from build123d import *

# Parameters (mm, degrees)
F0_R     = 175
F0_R_2   = 13
F1_DEPTH = 4


with BuildPart() as f1:
    # F0 (on Top) → F1 (new body)
    with BuildSketch(Plane.XY):
        Circle(F0_R)
        with Locations((-107.480231, -107.480231)):
            Circle(F0_R_2, mode=Mode.SUBTRACT)
        with Locations((-76, -131.635861)):
            Circle(F0_R_2, mode=Mode.SUBTRACT)
        with Locations((-39.340495, -146.820726)):
            Circle(F0_R_2, mode=Mode.SUBTRACT)
        with Locations((-45.922012, -110.865544)):
            Circle(F0_R_2, mode=Mode.SUBTRACT)
        with Locations((-73.051371, -95.202401)):
            Circle(F0_R_2, mode=Mode.SUBTRACT)
        with Locations((-15.663143, -118.973383)):
            Circle(F0_R_2, mode=Mode.SUBTRACT)
        with Locations((-131.635861, -76)):
            Circle(F0_R_2, mode=Mode.SUBTRACT)
        with Locations((-95.202401, -73.051371)):
            Circle(F0_R_2, mode=Mode.SUBTRACT)
        with Locations((-110.865544, -45.922012)):
            Circle(F0_R_2, mode=Mode.SUBTRACT)
        with Locations((-146.820726, -39.340495)):
            Circle(F0_R_2, mode=Mode.SUBTRACT)
        with Locations((-118.973383, -15.663143)):
            Circle(F0_R_2, mode=Mode.SUBTRACT)
        with Locations((0, -152)):
            Circle(F0_R_2, mode=Mode.SUBTRACT)
        with Locations((39.340495, -146.820726)):
            Circle(F0_R_2, mode=Mode.SUBTRACT)
        with Locations((76, -131.635861)):
            Circle(F0_R_2, mode=Mode.SUBTRACT)
        with Locations((15.663143, -118.973383)):
            Circle(F0_R_2, mode=Mode.SUBTRACT)
        with Locations((45.922012, -110.865544)):
            Circle(F0_R_2, mode=Mode.SUBTRACT)
        with Locations((73.051371, -95.202401)):
            Circle(F0_R_2, mode=Mode.SUBTRACT)
        with Locations((107.480231, -107.480231)):
            Circle(F0_R_2, mode=Mode.SUBTRACT)
        with Locations((95.202401, -73.051371)):
            Circle(F0_R_2, mode=Mode.SUBTRACT)
        with Locations((110.865544, -45.922012)):
            Circle(F0_R_2, mode=Mode.SUBTRACT)
        with Locations((131.635861, -76)):
            Circle(F0_R_2, mode=Mode.SUBTRACT)
        with Locations((118.973383, -15.663143)):
            Circle(F0_R_2, mode=Mode.SUBTRACT)
        with Locations((146.820726, -39.340495)):
            Circle(F0_R_2, mode=Mode.SUBTRACT)
        with Locations((-152, 0)):
            Circle(F0_R_2, mode=Mode.SUBTRACT)
        with Locations((-146.820726, 39.340495)):
            Circle(F0_R_2, mode=Mode.SUBTRACT)
        with Locations((-118.973383, 15.663143)):
            Circle(F0_R_2, mode=Mode.SUBTRACT)
        with Locations((-131.635861, 76)):
            Circle(F0_R_2, mode=Mode.SUBTRACT)
        with Locations((-110.865544, 45.922012)):
            Circle(F0_R_2, mode=Mode.SUBTRACT)
        with Locations((-95.202401, 73.051371)):
            Circle(F0_R_2, mode=Mode.SUBTRACT)
        with Locations((-107.480231, 107.480231)):
            Circle(F0_R_2, mode=Mode.SUBTRACT)
        with Locations((-73.051371, 95.202401)):
            Circle(F0_R_2, mode=Mode.SUBTRACT)
        with Locations((-45.922012, 110.865544)):
            Circle(F0_R_2, mode=Mode.SUBTRACT)
        with Locations((-15.663143, 118.973383)):
            Circle(F0_R_2, mode=Mode.SUBTRACT)
        with Locations((-76, 131.635861)):
            Circle(F0_R_2, mode=Mode.SUBTRACT)
        with Locations((-39.340495, 146.820726)):
            Circle(F0_R_2, mode=Mode.SUBTRACT)
        with Locations((118.973383, 15.663143)):
            Circle(F0_R_2, mode=Mode.SUBTRACT)
        with Locations((152, 0)):
            Circle(F0_R_2, mode=Mode.SUBTRACT)
        with Locations((146.820726, 39.340495)):
            Circle(F0_R_2, mode=Mode.SUBTRACT)
        with Locations((110.865544, 45.922012)):
            Circle(F0_R_2, mode=Mode.SUBTRACT)
        with Locations((95.202401, 73.051371)):
            Circle(F0_R_2, mode=Mode.SUBTRACT)
        with Locations((131.635861, 76)):
            Circle(F0_R_2, mode=Mode.SUBTRACT)
        with Locations((15.663143, 118.973383)):
            Circle(F0_R_2, mode=Mode.SUBTRACT)
        with Locations((73.051371, 95.202401)):
            Circle(F0_R_2, mode=Mode.SUBTRACT)
        with Locations((45.922012, 110.865544)):
            Circle(F0_R_2, mode=Mode.SUBTRACT)
        with Locations((0, 152)):
            Circle(F0_R_2, mode=Mode.SUBTRACT)
        with Locations((39.340495, 146.820726)):
            Circle(F0_R_2, mode=Mode.SUBTRACT)
        with Locations((76, 131.635861)):
            Circle(F0_R_2, mode=Mode.SUBTRACT)
        with Locations((107.480231, 107.480231)):
            Circle(F0_R_2, mode=Mode.SUBTRACT)
    extrude(amount=F1_DEPTH)


solid = f1.part
Geometry check sheet. Reference: the model listing, model coordinates, mm. Round coordinates to 2 decimals unless told otherwise and drop trailing zeros. Loops run counter-clockwise (first coordinate to the right, second up) from the corner with the lowest first, then second, coordinate; pieces in that order, holes last.
Item 1: Thickness scan on line 1 (Y direction, x = -136, z = 1.3); line 2 (X direction, y = 11.5, z = 2.9); line 3 (Y direction, x = -94, z = 2.25). Record the ranges inside material, lowest first.
Item 2: Cross-section at A-A on x = 69.5. Record the boundary of the cut face in (y, z), then the cut area to 3 significant figures.
Item 3: Gauge pin test, flat ends, axial feed: pin 1 (1.5 mm diameter, centred on y = 101, z = 2, fed in from +X); pin 2 (4 mm diameter, centred on x = 134, y = -50.5, fed in from -Z). Record the tip position at first contact, or that the pin passes through.
Item 4: Mould release check, pull along X, two halves, no side actions. Record for faces 1 (the cylindrical face through (-128.982, 118.273, 1.972)), 2 (the cylindrical face through (105.986, -15.092, 1.972)): pulls with the +X half, pulls with the -X half, needs draft (parallel to the pull), parting line crosses it, or undercut.
Item 5: Cross-section at C-C on z = 2.2. Count the separate pieces of the cut face and the enclosed holes in it, then the cut area to 3 significant figures.
Item 6: Cross-section at B-B on x = 152. Record the boundary of the cut face in (y, z).
Answer sheet:
1. line 1: y = -110.13 to -88.25, -63.75 to -46.55, -32.14 to 32.14, 46.55 to 63.75, 88.25 to 110.13
1. line 2: x = -174.62 to -158.06, -145.94 to -131.29, -106.66 to 106.66, 131.29 to 145.94, 158.06 to 174.62
1. line 3: y = -147.61 to -86, -60.11 to 60.11, 86 to 147.61
2. outline: (-160.61, 0) - (-142.89, 0) - (-142.89, 4) - (-160.61, 4) - close; (-120.38, 0) - (-107.71, 0) - (-107.71, 4) - (-120.38, 4) - close; (-82.7, 0) - (82.7, 0) - (82.7, 4) - (-82.7, 4) - close; (107.71, 0) - (120.38, 0) - (120.38, 4) - (107.71, 4) - close; (142.89, 0) - (160.61, 0) - (160.61, 4) - (142.89, 4) - close
2. area: 905 mm2
3. pin 1: stops at x = 143.44
3. pin 2: stops at z = 0
4. face 1: parting line crosses it
4. face 2: undercut
5. separate pieces: 1
5. enclosed holes: 48
5. area: 70,700 mm2
6. outline: (-86.72, 0) - (-51.26, 0) - (-51.26, 4) - (-86.72, 4) - close; (-27.42, 0) - (-13, 0) - (-13, 4) - (-27.42, 4) - close; (13, 0) - (27.42, 0) - (27.42, 4) - (13, 4) - close; (51.26, 0) - (86.72, 0) - (86.72, 4) - (51.26, 4) - close
